For this review, take the finished solid that the model builds, in its own axes (mm). Face numbers are marked on the shaded views. A direction names the side the tool comes from. Coordinates: 2 decimals unless noted, no trailing zeros. Write each loop counter-clockwise with the first axis right and the second up, starting at its lowest first coordinate (ties: lowest second). Pieces come first, ordered by that corner, then holes. Notation, with made-up numbers: (15, -16) -> (47, -16) arc R14 cw to (47, 4) -> close; hole circle Ø11 at (-27, 70). An arc over 180 degrees is marked (long way). One line per item, written item: value. Start each with the question number.
1) Add section A-A (z = 8). State the section outline as (x, y) points, and give its area (3 significant figures).
2) Add section B-B (y = 8). State the section outline as (x, z) points.
3) For probe 1 along Y at (x, z) = (0.75, -8); probe 2 along Z at (x, y) = (0.7, -8); probe 3 along Y at (x, z) = (1.2, 3), list the stretches that pass through material, from the lowest coordinate up. Write a range as from..to.
4) For pin 1 Ø5.5 at (y, z) = (-8, 8) entering from +X; pin 2 Ø3 at (y, z) = (8, -8) entering from +X, all flat-tipped, find the tip position at first contact; note any pin that passes through.
5) Mouldability with a two-part tool opening along Z and no side actions: class the marked faces 1, 2 and 3 as released by +Z, released by -Z, zero draft, split by the parting line, or undercut.
6) Machinability: for the marked faces 4 and 5, which of the approach directions +Z, -Z, +X, -X, +Y, -Y give a long, thin tool a straight path to every point of the face, cutting with its end or side? Answer none if there is none.
7) Add section C-C (x = 2.55). State the section outline as (y, z) points.
8) Add section D-D (y = -15.5). State the section outline as (x, z) points, and give its area (3 significant figures).
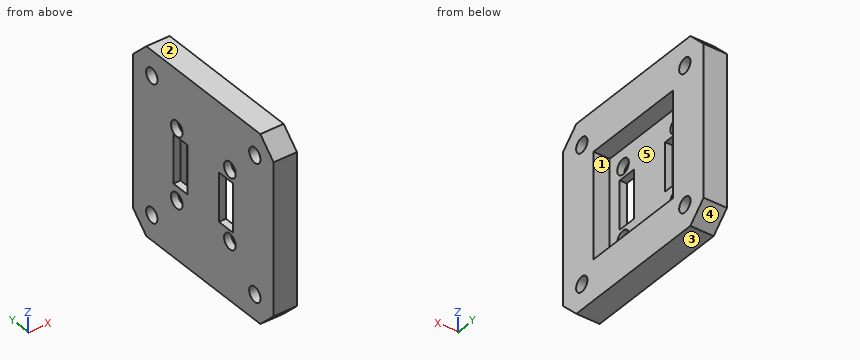
Autodesk Inventor part; units mm, degrees
ref_plane "YZ Plane" through (0, 0, 0) normal (1, 0, 0) x (0, 1, 0)
ref_plane "XZ Plane" through (0, 0, 0) normal (0, 1, 0) x (-1, 0, 0)
ref_plane "XY Plane" through (0, 0, 0) normal (0, 0, 1) x (1, 0, 0)
sketch "Skizze1" plane through (0, 0, 0) normal (1, 0, 0) x (0, 1, 0)
  line L0 (-21.15, -21.15) -> (21.15, -21.15)
  line L1 (21.15, -21.15) -> (21.15, 21.15)
  line L2 (21.15, 21.15) -> (-21.15, 21.15)
  line L3 (-21.15, 21.15) -> (-21.15, -21.15)
  line L4 (-21.15, -21.15) -> (21.15, 21.15) construction
  line L5 (21.15, -21.15) -> (-21.15, 21.15) construction
  point P0 (0, 0)
  dimension "d0" = 42.3
  dimension "d1" = 42.3
extrude "Extrusion1" add sketch "Skizze1" along normal blind 5.3
sketch "Skizze2" plane through (5.3, 0, 0) normal (1, 0, 0) x (0, 0, -1)
  line L0 (12, -12) -> (-12, -12)
  line L1 (-12, -12) -> (-12, 12)
  line L2 (-12, 12) -> (12, 12)
  line L3 (12, 12) -> (12, -12)
  line L4 (12, -12) -> (-12, 12) construction
  line L5 (-12, -12) -> (12, 12) construction
  point P0 (0, 0)
  dimension "d4" = 24
  dimension "d5" = 24
extrude "Extrusion2" cut sketch "Skizze2" against normal blind 3.7
sketch "Skizze3" plane through (1.6, 0, 0) normal (1, 0, 0) x (0, 0, -1)
  point P0 (0, 0)
  point P1 (-8, 8)
  point P2 (8, 8)
  point P3 (8, -8)
  point P4 (-8, -8)
  dimension "d16" = 8
  dimension "d17" = 8
  dimension "d18" = 8
  dimension "d19" = 8
  dimension "d20" = 8
  dimension "d21" = 8
  dimension "d22" = 8
  dimension "d23" = 8
hole "Bohrung1" at (1.6, 8, 8) at (1.6, 8, -8) at (1.6, -8, -8) at (1.6, -8, 8) direction (-1, 0, 0) diameter 3.5 end through all
sketch "Skizze4" plane through (5.3, 0, 0) normal (1, 0, 0) x (0, 0, -1)
  point P0 (0, 0)
  point P1 (-15.5, 15.5)
  point P2 (15.5, 15.5)
  point P3 (15.5, -15.5)
  point P4 (-15.5, -15.5)
  dimension "d31" = 15.5
  dimension "d32" = 15.5
  dimension "d33" = 15.5
  dimension "d34" = 15.5
  dimension "d35" = 15.5
  dimension "d36" = 15.5
  dimension "d37" = 15.5
  dimension "d38" = 15.5
hole "Bohrung2" at (5.3, 15.5, 15.5) at (5.3, 15.5, -15.5) at (5.3, -15.5, -15.5) at (5.3, -15.5, 15.5) direction (-1, 0, 0) diameter 3.4 end through all
chamfer "Fase1" distance 4 angle 45 4 edges at (2.65, -21.15, -21.15) (2.65, -21.15, 21.15) (2.65, 21.15, -21.15) (2.65, 21.15, 21.15)
sketch "Skizze5" plane through (1.6, 0, 0) normal (1, 0, 0) x (0, 0, -1)
  line L0 (-6.2, 9) -> (4.8, 9)
  line L1 (4.8, 9) -> (4.8, 4.7)
  line L2 (4.8, 4.7) -> (-6.2, 4.7)
  line L3 (-6.2, 4.7) -> (-6.2, 9)
  line L4 (-12, 12) -> (12, 12)
  line L5 (-12, -12) -> (-12, 12)
  point P0 (0, 0)
  point P1 (-6.2, 6.85)
  dimension "d42" = 11
  dimension "d43" = 4.3
  dimension "d44" = 3
  dimension "d45" = 5.8
sketch "Skizze6" plane through (1.6, 0, 0) normal (1, 0, 0) x (0, 0, -1)
  line L0 (-5.5, -4.7) -> (5.5, -4.7)
  line L1 (5.5, -4.7) -> (5.5, -9)
  line L2 (5.5, -9) -> (-5.5, -9)
  line L3 (-5.5, -9) -> (-5.5, -4.7)
  line L4 (12, -12) -> (-12, -12)
  point P0 (0, 0)
  dimension "d46" = 11
  dimension "d47" = 4.3
  dimension "d48" = 3
  dimension "d49" = 5.5
extrude "Extrusion3" cut sketch "Skizze5" against normal blind 10
extrude "Extrusion4" cut sketch "Skizze6" against normal blind 10
properties part number "EncoderHalter"
Numbers:
1. outline: (0, -21.15) -> (5.3, -21.15) -> (5.3, -12) -> (1.6, -12) -> (1.6, -9.75) -> (0, -9.75) -> close; (0, -6.25) -> (1.6, -6.25) -> (1.6, 6.25) -> (0, 6.25) -> close; (0, 9.75) -> (1.6, 9.75) -> (1.6, 12) -> (5.3, 12) -> (5.3, 21.15) -> (0, 21.15) -> close
1. area: 124 mm²
2. outline: (0, -21.15) -> (5.3, -21.15) -> (5.3, -12) -> (1.6, -12) -> (1.6, -9.75) -> (0, -9.75) -> close; (0, -6.25) -> (1.6, -6.25) -> (1.6, -4.8) -> (0, -4.8) -> close; (0, 6.2) -> (1.6, 6.2) -> (1.6, 6.25) -> (0, 6.25) -> close; (0, 9.75) -> (1.6, 9.75) -> (1.6, 12) -> (5.3, 12) -> (5.3, 21.15) -> (0, 21.15) -> close
3. probe 1: -21.15..-9.75, -6.25..6.25, 9.75..21.15
3. probe 2: -21.15..-9.75, -6.25..-5.5, 5.5..6.25, 9.75..21.15
3. probe 3: -21.15..-9, -4.7..4.7, 9..21.15
4. pin 1: x = 1.6
4. pin 2: through
5. face 1: undercut
5. face 2: released by +Z
5. face 3: released by -Z
6. face 4: -Z, +X, -X, +Y
6. face 5: +X
7. outline: (-21.15, -17.15) -> (-17.15, -21.15) -> (17.15, -21.15) -> (21.15, -17.15) -> (21.15, 17.15) -> (17.15, 21.15) -> (-17.15, 21.15) -> (-21.15, 17.15) -> close; hole circle Ø3.4 at (-15.5, -15.5); hole circle Ø3.4 at (-15.5, 15.5); hole (-12, -12) -> (12, -12) -> (12, 12) -> (-12, 12) -> close; hole circle Ø3.4 at (15.5, -15.5); hole circle Ø3.4 at (15.5, 15.5)
8. outline: (0, -21.15) -> (5.3, -21.15) -> (5.3, -17.2) -> (0, -17.2) -> close; (0, -13.8) -> (5.3, -13.8) -> (5.3, 13.8) -> (0, 13.8) -> close; (0, 17.2) -> (5.3, 17.2) -> (5.3, 21.15) -> (0, 21.15) -> close
8. area: 188 mm²
